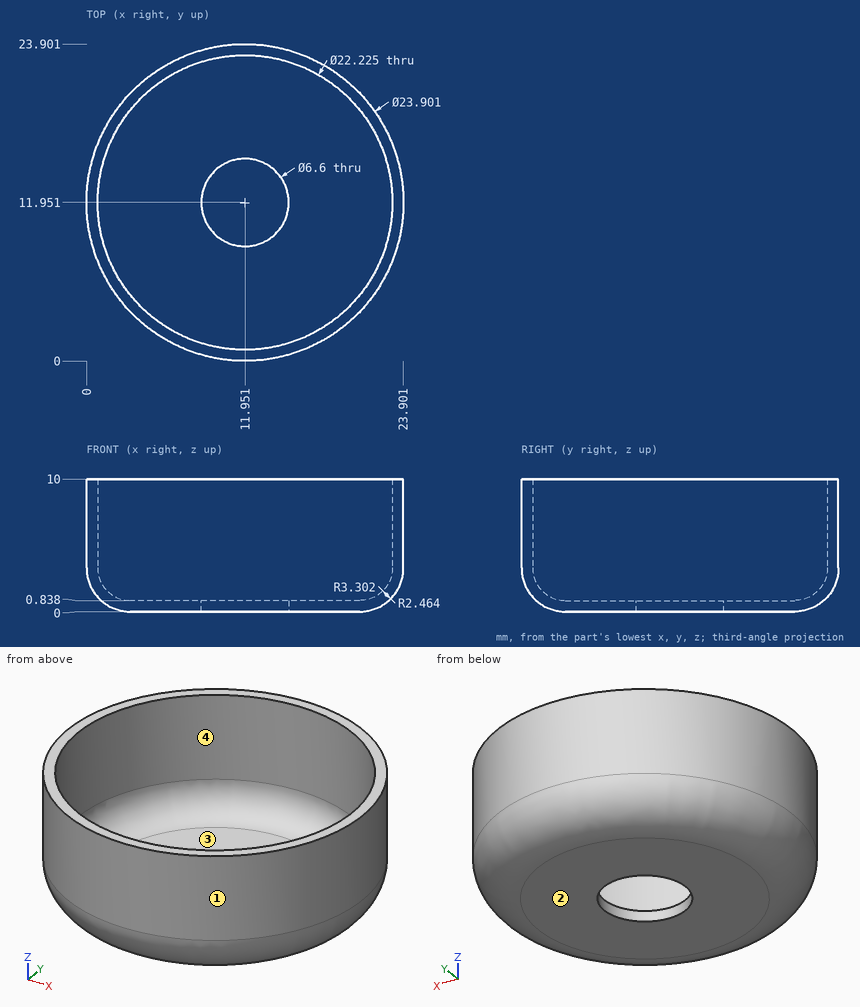
Print and shaded views of the part. All mm, measured from the part's lowest x, y and z. Round coordinates to 2 decimals unless told otherwise and drop trailing zeros. Answer in a Markdown table with one row per item. Add a question column.
Item 1: Drill centre lines: line 1 (Z direction, x = 14.25, y = 18); line 2 (Y direction, x = 12, z = 5.75); line 3 (X direction, y = 5, z = 5.75). Where is each one in solid material? Low to high. Write a range as from..to.
Item 2: Mould opens along Y. For the marked faces 1, 2, 3 and 4 say: pulls with the +Y half, pulls with the -Y half, needs draft (parallel to the pull), parting line crosses it, or undercut.
Item 3: Drop flat-ended pins along their axis: pin 1 Ø6 at (x, z) = (18, 5.5) entering from +Y; pin 2 Ø2 at (x, z) = (15, 5.5) entering from +Y (1 decimal); pin 3 Ø6 at (x, y) = (17.5, 9) entering from +Z. Give the stop position or say it passes through.
Findings below:
| question | item | result |
|---|---|---|
| 1 | line 1 | z = 0..0.84 |
| 1 | line 2 | y = 0..0.84, 23.06..23.9 |
| 1 | line 3 | x = 2.23..3.28, 20.62..21.67 |
| 2 | face 1 | parting line crosses it |
| 2 | face 2 | needs draft |
| 2 | face 3 | undercut |
| 2 | face 4 | undercut |
| 3 | pin 1 | stops at y = 23.51 |
| 3 | pin 2 | stops at y = 23.7 |
| 3 | pin 3 | stops at z = 0.92 |
